from build123d import *

# Parameters (mm, degrees)
BOSS_EXTRUDE1_DEPTH      = 80
SKETCH2_W                = 60
SKETCH2_H                = 28
CUT_EXTRUDE1_DEPTH       = 80
SKETCH3_W                = 39.904961116
SKETCH3_H                = 80
BOSS_EXTRUDE2_DEPTH      = 70
CUT_EXTRUDE4_REACH       = 115.545
SKETCH6_W                = 24.904961116
SKETCH6_H                = 60
CUT_EXTRUDE5_DEPTH       = 70
SKETCH7_W                = 10
SKETCH7_H                = 4
BOSS_EXTRUDE3_DEPTH      = 13
SKETCH8_R                = 3.1
CUT_EXTRUDE6_DEPTH       = 1
CHAMFER1_SIZE            = 1
CHAMFER2_SIZE            = 3
CHAMFER2_OF_MIRROR1_SIZE = 3
SKETCH9_W                = 10
SKETCH9_H                = 4
BOSS_EXTRUDE4_DEPTH      = 13
SKETCH10_R               = 3.1
CUT_EXTRUDE7_DEPTH       = 1
CHAMFER3_SIZE            = 3
CHAMFER4_SIZE            = 1
CHAMFER5_SIZE            = 1
CUT_EXTRUDE8_REACH       = 125.05


with BuildPart() as part:
    # Sketch1 → Boss-Extrude1 (new body)
    with BuildSketch(Plane.XY):
        Polygon((9, 36), (39.904961116, 17.536972664), (39.904961116, 0), (0, 0), (0, 36), align=None)
    extrude(amount=BOSS_EXTRUDE1_DEPTH)

    # Sketch2 → Cut-Extrude1 (cut)
    with BuildSketch(Plane.ZY):
        with Locations((40, 22)):
            Rectangle(SKETCH2_W, SKETCH2_H)
    extrude(amount=-CUT_EXTRUDE1_DEPTH, mode=Mode.SUBTRACT)

    # Sketch3 → Boss-Extrude2 (add)
    with BuildSketch(Plane.XZ):
        with Locations((19.952480558, 40)):
            Rectangle(SKETCH3_W, SKETCH3_H)
    extrude(amount=BOSS_EXTRUDE2_DEPTH)

    # Sketch4 → Cut-Extrude4 (cut, up to next)
    with BuildSketch(Plane(origin=(39.904961116, 0, 0), x_dir=(0, 0, -1), z_dir=(1, 0, 0)), mode=Mode.PRIVATE) as cut_extrude4_sk1:
        Polygon((-10, 8), (-40, -7.119896394), (-70, 8), align=None)
    cut_extrude4_tool1 = extrude(cut_extrude4_sk1.sketch, amount=-CUT_EXTRUDE4_REACH, mode=Mode.PRIVATE) & part.part
    # Sketch4 → Cut-Extrude4 (cut, up to next)
    with BuildSketch(Plane(origin=(39.904961116, 0, 0), x_dir=(0, 0, -1), z_dir=(1, 0, 0)), mode=Mode.PRIVATE) as cut_extrude4_sk2:
        Polygon((-47.440527175, -10.869896394), (-70, 0.5), (-70, -22.239792788), align=None)
    cut_extrude4_tool2 = extrude(cut_extrude4_sk2.sketch, amount=-CUT_EXTRUDE4_REACH, mode=Mode.PRIVATE) & part.part
    # Sketch4 → Cut-Extrude4 (cut, up to next)
    with BuildSketch(Plane(origin=(39.904961116, 0, 0), x_dir=(0, 0, -1), z_dir=(1, 0, 0)), mode=Mode.PRIVATE) as cut_extrude4_sk3:
        Polygon((-47.440527175, -41.130103606), (-70, -29.760207212), (-70, -52.5), align=None)
    cut_extrude4_tool3 = extrude(cut_extrude4_sk3.sketch, amount=-CUT_EXTRUDE4_REACH, mode=Mode.PRIVATE) & part.part
    # Sketch4 → Cut-Extrude4 (cut, up to next)
    with BuildSketch(Plane(origin=(39.904961116, 0, 0), x_dir=(0, 0, -1), z_dir=(1, 0, 0)), mode=Mode.PRIVATE) as cut_extrude4_sk4:
        Polygon((-10, -60), (-40, -44.880103606), (-70, -60), align=None)
    cut_extrude4_tool4 = extrude(cut_extrude4_sk4.sketch, amount=-CUT_EXTRUDE4_REACH, mode=Mode.PRIVATE) & part.part
    # Sketch4 → Cut-Extrude4 (cut, up to next)
    with BuildSketch(Plane(origin=(39.904961116, 0, 0), x_dir=(0, 0, -1), z_dir=(1, 0, 0)), mode=Mode.PRIVATE) as cut_extrude4_sk5:
        Polygon((-10, -52.5), (-10, -29.760207212), (-32.559472825, -41.130103606), align=None)
    cut_extrude4_tool5 = extrude(cut_extrude4_sk5.sketch, amount=-CUT_EXTRUDE4_REACH, mode=Mode.PRIVATE) & part.part
    # Sketch4 → Cut-Extrude4 (cut, up to next)
    with BuildSketch(Plane(origin=(39.904961116, 0, 0), x_dir=(0, 0, -1), z_dir=(1, 0, 0)), mode=Mode.PRIVATE) as cut_extrude4_sk6:
        Polygon((-62.579725368, -26), (-40, -14.619896394), (-17.420274632, -26), (-40, -37.380103606), align=None)
    cut_extrude4_tool6 = extrude(cut_extrude4_sk6.sketch, amount=-CUT_EXTRUDE4_REACH, mode=Mode.PRIVATE) & part.part
    # Sketch4 → Cut-Extrude4 (cut, up to next)
    with BuildSketch(Plane(origin=(39.904961116, 0, 0), x_dir=(0, 0, -1), z_dir=(1, 0, 0)), mode=Mode.PRIVATE) as cut_extrude4_sk7:
        Polygon((-10, -22.239792788), (-10, 0.5), (-32.559472825, -10.869896394), align=None)
    cut_extrude4_tool7 = extrude(cut_extrude4_sk7.sketch, amount=-CUT_EXTRUDE4_REACH, mode=Mode.PRIVATE) & part.part
    add(cut_extrude4_tool1.solids().sort_by_distance((39.904961, 2.960035, 40))[0], mode=Mode.SUBTRACT)
    add(cut_extrude4_tool2.solids().sort_by_distance((39.904961, -10.869896, 62.480176))[0], mode=Mode.SUBTRACT)
    add(cut_extrude4_tool3.solids().sort_by_distance((39.904961, -41.130104, 62.480176))[0], mode=Mode.SUBTRACT)
    add(cut_extrude4_tool4.solids().sort_by_distance((39.904961, -54.960035, 40))[0], mode=Mode.SUBTRACT)
    add(cut_extrude4_tool5.solids().sort_by_distance((39.904961, -41.130104, 17.519824))[0], mode=Mode.SUBTRACT)
    add(cut_extrude4_tool6.solids().sort_by_distance((39.904961, -26, 40))[0], mode=Mode.SUBTRACT)
    add(cut_extrude4_tool7.solids().sort_by_distance((39.904961, -10.869896, 17.519824))[0], mode=Mode.SUBTRACT)

    # Sketch6 → Cut-Extrude5 (cut)
    with BuildSketch(Plane(origin=(0, 8, 0), x_dir=(1, 0, 0), z_dir=(0, 1, 0))):
        with Locations((19.952480558, -40)):
            Rectangle(SKETCH6_W, SKETCH6_H)
    extrude(amount=-CUT_EXTRUDE5_DEPTH, mode=Mode.SUBTRACT)

    # Sketch7 → Boss-Extrude3 (add)
    with BuildSketch(Plane(origin=(0, 0, 0), x_dir=(-1, 0, 0), z_dir=(0, 0, -1))):
        with Locations((-34.904961116, -68)):
            Rectangle(SKETCH7_W, SKETCH7_H)
    boss_extrude3 = extrude(amount=BOSS_EXTRUDE3_DEPTH)

    # Sketch8 → Cut-Extrude6 (cut)
    with BuildSketch(Plane(origin=(0, -66, 0), x_dir=(1, 0, 0), z_dir=(0, 1, 0))):
        with Locations(Location((34.904961116, 5, 0), (0, 0, 270))):
            Circle(SKETCH8_R)
    cut_extrude6 = extrude(amount=-CUT_EXTRUDE6_DEPTH, mode=Mode.SUBTRACT)

    # Chamfer1
    chamfer1_edges = [part.edges().sort_by_distance(p)[0] for p in [
        (34.904961116, -67, -8.1),
    ]]
    chamfer(chamfer1_edges, length=CHAMFER1_SIZE - 0.0001)  # a hair under: the kernel refuses the full size

    # Chamfer2
    chamfer2_edges = [part.edges().sort_by_distance(p)[0] for p in [
        (34.904961116, -66, -13),
    ]]
    chamfer(chamfer2_edges, length=CHAMFER2_SIZE)

    # Mirror1: Boss-Extrude3, Cut-Extrude6 across plane
    add(boss_extrude3.mirror(Plane.XY.offset(40)))
    add(cut_extrude6.mirror(Plane.XY.offset(40)), mode=Mode.SUBTRACT)

    # Chamfer2 of Mirror1
    chamfer2_of_mirror1_edges = [part.edges().sort_by_distance(p)[0] for p in [
        (34.904961116, -66, 93),
    ]]
    chamfer(chamfer2_of_mirror1_edges, length=CHAMFER2_OF_MIRROR1_SIZE)

    # Sketch9 → Boss-Extrude4 (add)
    with BuildSketch(Plane.ZY):
        with Locations((40, -68)):
            Rectangle(SKETCH9_W, SKETCH9_H)
    extrude(amount=BOSS_EXTRUDE4_DEPTH)

    # Sketch10 → Cut-Extrude7 (cut)
    with BuildSketch(Plane(origin=(0, -66, 0), x_dir=(1, 0, 0), z_dir=(0, 1, 0))):
        with Locations(Location((-5, -40, 0), (0, 0, 270))):
            Circle(SKETCH10_R)
    extrude(amount=-CUT_EXTRUDE7_DEPTH, mode=Mode.SUBTRACT)

    # Chamfer3
    chamfer3_edges = [part.edges().sort_by_distance(p)[0] for p in [
        (-13, -66, 40),
    ]]
    chamfer(chamfer3_edges, length=CHAMFER3_SIZE)

    # Chamfer4
    chamfer4_edges = [part.edges().sort_by_distance(p)[0] for p in [
        (-5, -67, 36.9),
    ]]
    chamfer(chamfer4_edges, length=CHAMFER4_SIZE - 0.0001)  # a hair under: the kernel refuses the full size

    # Chamfer5
    chamfer5_edges = [part.edges().sort_by_distance(p)[0] for p in [
        (34.904961116, -67, 88.1),
    ]]
    chamfer(chamfer5_edges, length=CHAMFER5_SIZE - 0.0001)  # a hair under: the kernel refuses the full size

    # Sketch11 → Cut-Extrude8 (cut, up to next)
    with BuildSketch(Plane.XY.offset(80), mode=Mode.PRIVATE) as cut_extrude8_sk1:
        Polygon((0, 17.536972664), (0, 36), (9, 36), (24.289010788, 26.866145307), (24.289010788, 17.536972664), align=None)
    cut_extrude8_tool1 = extrude(cut_extrude8_sk1.sketch, amount=-CUT_EXTRUDE8_REACH, mode=Mode.PRIVATE) & part.part
    add(cut_extrude8_tool1.solids().sort_by_distance((10.844723, 25.627535, 80))[0], mode=Mode.SUBTRACT)


solid = part.part
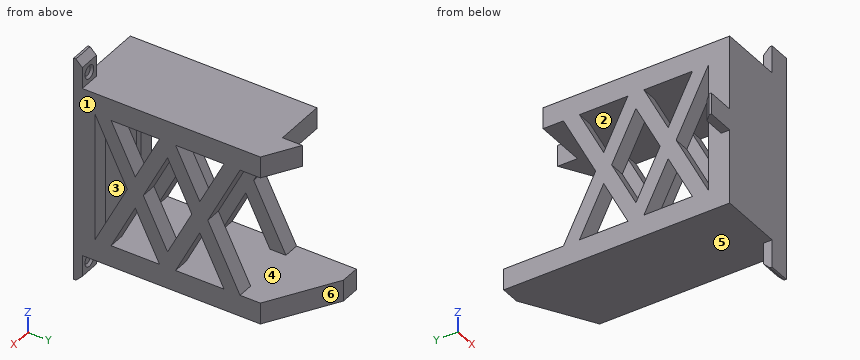
CAD build for the part. Positions are in the model's coordinates, mm. Face numbers are marked on the shaded views. A direction names the side the tool comes from. Round coordinates to 2 decimals unless told otherwise and drop trailing zeros. Write each loop counter-clockwise with the first axis right and the second up, starting at its lowest first coordinate (ties: lowest second). Pieces come first, ordered by that corner, then holes.
(1) 3-axis set-ups, long thin cutter, end or side, ignore diameter. For the marked faces 1, 2 and 3: which of +Z, -Z, +X, -X, +Y, -Y reach the whole face in a straight line?
(2) Drop flat-ended pins along their axis: P1, Ø1, axis at x = -1.5, y = -49.5, coming from the +Z side; P2, Ø6, axis at x = 2, z = 51.5, coming from the +Y side; P3, Ø3, axis at y = -67, z = -9.5, coming from the -X side; P4, Ø1.6, axis at y = -61, z = 25, coming from the -X side. Give the stop position or say it passes through.
(3) Slice it at C-C, the plane y = -50.5. Write the cut outline in (x, z), and give its area (3 significant figures).
(4) Mould opens along Z. For the marked faces 4, 5 and 6 say: pulls with the +Z half, pulls with the -Z half, needs draft (parallel to the pull), parting line crosses it, or undercut.
(5) Probe line 1 along Z through (x, y) = (12.5, -17); line 2 along Z through (x, y) = (1, -44); line 3 along Y through (x, z) = (27.5, 55). List the from-to ranges inside material, lowest first.
(6) Slice it at A-A, the plane y = 10.5. Write the cut outline in (x, z).
From the geometry:
1. face 1: +Z, -Z, +X, +Y, -Y
1. face 2: none
1. face 3: +Y
2. P1: passes through
2. P2: stops at y = 0.19
2. P3: stops at x = 29.9
2. P4: stops at x = 0
3. outline: (0, 0) - (39.9, 0) - (39.9, 10) - (0, 10) - close; (0, 13.97) - (7.5, 13.97) - (7.5, 28.85) - (0, 28.85) - close; (0, 51.15) - (7.5, 51.15) - (7.5, 66.03) - (0, 66.03) - close; (0, 70) - (39.9, 70) - (39.9, 80) - (0, 80) - close; (32.4, 13.97) - (39.9, 13.97) - (39.9, 28.85) - (32.4, 28.85) - close; (32.4, 51.15) - (39.9, 51.15) - (39.9, 66.03) - (32.4, 66.03) - close
3. area: 1,240 mm2
4. face 4: undercut
4. face 5: pulls with the -Z half
4. face 6: needs draft
5. line 1: z = 0 to 10, 70 to 80
5. line 2: z = 0 to 10, 26.87 to 53.13, 70 to 80
5. line 3: y = -70 to -62
6. outline: (0, 0) - (39.9, 0) - (39.9, 10) - (0, 10) - close; (0, 70) - (39.9, 70) - (39.9, 80) - (0, 80) - close
